Design review of the part built by this model. Coordinates are the model's own, in mm. A direction names the side the tool comes from. Coordinates: 2 decimals unless noted, no trailing zeros. Loops run counter-clockwise (first coordinate to the right, second up) from the corner with the lowest first, then second, coordinate; pieces in that order, holes last. Notation, with made-up numbers: (-11.75, 17) -> (43.25, 17) arc R12 ccw to (43.25, 37) -> close; hole circle Ø6 at (-30, 67.5). An arc over 180 degrees is marked (long way). One line per item, written item: value. Start each with the question number.
1. Draft analysis for pull direction Z (two halves, no side actions). For faces 1 (the flat face through (2, 9, 0)), 2 (the flat face through (5.3, 18.5, 28)), 3 (the flat face through (-3, 18.5, -5.1)), state which applies: pulls with the +Z half, pulls with the -Z half, needs draft (parallel to the pull), parting line crosses it, or undercut.
2. Insertion check: pin 1 (1.9 mm diameter, centred on x = 2.5, y = 12.5, fed in from +Z); pin 2 (8 mm diameter, centred on y = 7, z = 15, fed in from +X); pin 3 (3 mm diameter, centred on x = 1.5, z = -5, fed in from -Y). Each pin has a flat end and moves straight along its axis. Give the tip position at first contact, or say it passes through.
3. For probe 1 along Z at (x, y) = (2.25, 15.5); probe 2 along X at (y, z) = (17, 7); probe 3 along Y at (x, z) = (-1.5, 32), list the stretches that pass through material, from the lowest coordinate up.
4. Add section A-A on x = -1. Write out the cut boundary in (y, z), plus the area to 3 significant figures.
5. Add section D-D on y = 5.5. Write out the cut boundary in (x, z).
6. Add section C-C on x = 1.5. Write out the cut boundary in (y, z).
7. Add section B-B on z = 20.5. Write out the cut boundary in (x, y).
8. Machinability: for faces 4 (the flat face through (-1.5, 18.5, 28)), 5 (the flat face through (2, 18, -5)), 6 (the flat face through (2, 18, 33)), 7 (the flat face through (2, 2, 14)), 8 (the flat face through (5.3, 18.5, 0)), which of the approach directions +Z, -Z, +X, -X, +Y, -Y give a long, thin tool a straight path to every point of the face, cutting with its end or side? Answer none if there is none.
```python
from build123d import *

# Parameters (mm, degrees)
BOSS_EXTRUDE2_DEPTH = 28
SKETCH3_W           = 3.8
SKETCH3_H           = 1
BOSS_EXTRUDE3_DEPTH = 10
SKETCH4_W           = 3.8
SKETCH4_H           = 1
BOSS_EXTRUDE4_DEPTH = 10
SKETCH5_W           = 10
SKETCH5_H           = 1
BOSS_EXTRUDE5_DEPTH = 3
SKETCH6_W           = 10
SKETCH6_H           = 1
BOSS_EXTRUDE6_DEPTH = 3
SKETCH7_W           = 10
SKETCH7_H           = 1
BOSS_EXTRUDE7_DEPTH = 3
SKETCH8_W           = 10
SKETCH8_H           = 1
BOSS_EXTRUDE8_DEPTH = 3


with BuildPart() as part:
    # Sketch1 → Boss-Extrude2 (new body)
    with BuildSketch(Plane.XY):
        Polygon((2.8, 0), (3.8, 0), (3.8, 19), (0, 19), (0, 0), (0.995254582, 0), (0.995254582, 2), (2.8, 2), align=None)
    extrude(amount=BOSS_EXTRUDE2_DEPTH)

    # Sketch3 → Boss-Extrude3 (add)
    with BuildSketch(Plane.XY.offset(28)):
        with Locations((1.9, 18.5)):
            Rectangle(SKETCH3_W, SKETCH3_H)
    extrude(amount=BOSS_EXTRUDE3_DEPTH)

    # Sketch4 → Boss-Extrude4 (add)
    with BuildSketch(Plane(origin=(0, 0, 0), x_dir=(-1, 0, 0), z_dir=(0, 0, -1))):
        with Locations((-1.9, 18.5)):
            Rectangle(SKETCH4_W, SKETCH4_H)
    extrude(amount=BOSS_EXTRUDE4_DEPTH)

    # Sketch5 → Boss-Extrude5 (add)
    with BuildSketch(Plane(origin=(3.8, 0, 0), x_dir=(0, 0, -1), z_dir=(1, 0, 0))):
        with Locations((5, 18.5)):
            Rectangle(SKETCH5_W, SKETCH5_H)
    extrude(amount=BOSS_EXTRUDE5_DEPTH)

    # Sketch6 → Boss-Extrude6 (add)
    with BuildSketch(Plane.ZY):
        with Locations((-5, 18.5)):
            Rectangle(SKETCH6_W, SKETCH6_H)
    extrude(amount=BOSS_EXTRUDE6_DEPTH)

    # Sketch7 → Boss-Extrude7 (add)
    with BuildSketch(Plane.ZY):
        with Locations((33, 18.5)):
            Rectangle(SKETCH7_W, SKETCH7_H)
    extrude(amount=BOSS_EXTRUDE7_DEPTH)

    # Sketch8 → Boss-Extrude8 (add)
    with BuildSketch(Plane(origin=(3.8, 0, 0), x_dir=(0, 0, -1), z_dir=(1, 0, 0))):
        with Locations((-33, 18.5)):
            Rectangle(SKETCH8_W, SKETCH8_H)
    extrude(amount=BOSS_EXTRUDE8_DEPTH)


solid = part.part
```
Worked answers:
1. face 1: pulls with the -Z half
1. face 2: undercut
1. face 3: needs draft
2. pin 1: stops at z = 28
2. pin 2: stops at x = 3.8
2. pin 3: stops at y = 18
3. probe 1: z = 0 to 28
3. probe 2: x = 0 to 3.8
3. probe 3: y = 18 to 19
4. outline: (18, -10) -> (19, -10) -> (19, 0) -> (18, 0) -> close; (18, 28) -> (19, 28) -> (19, 38) -> (18, 38) -> close
4. area: 20.0 mm²
5. outline: (0, 0) -> (3.8, 0) -> (3.8, 28) -> (0, 28) -> close
6. outline: (2, 0) -> (18, 0) -> (18, -10) -> (19, -10) -> (19, 38) -> (18, 38) -> (18, 28) -> (2, 28) -> close
7. outline: (0, 0) -> (1, 0) -> (1, 2) -> (2.8, 2) -> (2.8, 0) -> (3.8, 0) -> (3.8, 19) -> (0, 19) -> close
8. face 4: -X, +Y, -Y
8. face 5: -Z, +X, -X, -Y
8. face 6: +Z, +X, -X, -Y
8. face 7: +Z, -Z, -Y
8. face 8: +X, +Y, -Y
